For this review, take the finished solid that the model builds, in its own axes (mm). Round coordinates to 2 decimals unless told otherwise and drop trailing zeros. Order: outer loops, then holes, each group sorted by start corner. A loop starts at its lowest first (then second) coordinate and runs counter-clockwise, first axis right, second up. Notation, with made-up numbers: M 3,67 L 57,67 A8 cw 57,77 Z; hole C 16,13 d2. An arc over 180 degrees is marked long. Put each result on its own line as item: value.
from build123d import *

# Parameters (mm, degrees)
SKETCH_8_W           = 73
SKETCH_8_H           = 92
EXTRUDE_5_DEPTH      = 12
SKETCH_9_W           = 71
SKETCH_9_H           = 90
CUT_EXTRUDE_3_DEPTH  = 10
SKETCH_11_W          = 73
SKETCH_11_H          = 6
EXTRUDE_8_DEPTH      = 7
SKETCH_12_W          = 4
SKETCH_12_H          = 19
EXTRUDE_10_DEPTH     = 7
SKETCH_13_W          = 4
SKETCH_13_H          = 21
EXTRUDE_13_DEPTH     = 7
SKETCH_14_W          = 7
SKETCH_14_H          = 12
EXTRUDE_14_DEPTH     = 7
SKETCH_15_W          = 7
SKETCH_15_H          = 58
EXTRUDE_15_DEPTH     = 7
SKETCH_17_W          = 40
SKETCH_17_H          = 6
EXTRUDE_16_DEPTH     = 7
SKETCH_18_W          = 20
SKETCH_18_H          = 5
EXTRUDE_17_DEPTH     = 7
SKETCH_19_W          = 16
SKETCH_19_H          = 4
EXTRUDE_18_DEPTH     = 7
SKETCH_20_W          = 4
SKETCH_20_H          = 7
EXTRUDE_19_DEPTH     = 7
SKETCH_21_W          = 5
SKETCH_21_H          = 31
EXTRUDE_22_DEPTH     = 5
SKETCH_23_W          = 9
SKETCH_23_H          = 12
EXTRUDE_23_DEPTH     = 7
SKETCH_24_W          = 17
SKETCH_24_H          = 10
EXTRUDE_24_DEPTH     = 7
SKETCH_25_W          = 8
SKETCH_25_H          = 4
EXTRUDE_25_DEPTH     = 7
SKETCH_28_W          = 8
SKETCH_28_H          = 31
EXTRUDE_26_DEPTH     = 5
SKETCH_32_W          = 10
SKETCH_32_H          = 1
CUT_EXTRUDE_4_DEPTH  = 5
SKETCH_33_W          = 8
SKETCH_33_H          = 51
EXTRUDE_27_DEPTH     = 5
SKETCH_35_W          = 10
SKETCH_35_H          = 1
EXTRUDE_28_DEPTH     = 10
SKETCH_37_W          = 11
SKETCH_37_H          = 1
CUT_EXTRUDE_7_DEPTH  = 1
SKETCH_39_W          = 11
SKETCH_39_H          = 1
CUT_EXTRUDE_8_DEPTH  = 1
SKETCH_40_W          = 1
SKETCH_40_H          = 1
EXTRUDE_29_DEPTH     = 7
SKETCH_41_R          = 1
CUT_EXTRUDE_9_DEPTH  = 9
EXTRUDE_30_DEPTH     = 4
SKETCH_44_W          = 4
SKETCH_44_H          = 6
SKETCH_44_W_2        = 3
SKETCH_44_H_2        = 5
SKETCH_44_H_3        = 7
SKETCH_44_W_3        = 7
SKETCH_44_H_4        = 7.504780259
EXTRUDE_31_DEPTH     = 7
SKETCH_45_W          = 73
SKETCH_45_H          = 1
CUT_EXTRUDE_10_DEPTH = 100
SKETCH_47_W          = 73
SKETCH_47_H          = 1
CUT_EXTRUDE_11_DEPTH = 100


with BuildPart() as part:
    # 草图8 → 凸台-拉伸5 (new body)
    with BuildSketch(Plane(origin=(0, 0, 0), x_dir=(1, 0, 0), z_dir=(0, 1, 0))):
        with Locations((36.5, 46)):
            Rectangle(SKETCH_8_W, SKETCH_8_H)
    extrude(amount=EXTRUDE_5_DEPTH)

    # 草图9 → 切除-拉伸3 (cut)
    with BuildSketch(Plane(origin=(0, 12, 0), x_dir=(1, 0, 0), z_dir=(0, 1, 0))):
        with Locations((36.5, 46)):
            Rectangle(SKETCH_9_W, SKETCH_9_H)
    extrude(amount=-CUT_EXTRUDE_3_DEPTH, mode=Mode.SUBTRACT)

    # 草图11 → 凸台-拉伸8 (add)
    with BuildSketch(Plane(origin=(0, 0, 0), x_dir=(1, 0, 0), z_dir=(0, 1, 0))):
        with Locations((36.5, 89)):
            Rectangle(SKETCH_11_W, SKETCH_11_H)
    extrude(amount=EXTRUDE_8_DEPTH)

    # 草图12 → 凸台-拉伸10 (add)
    with BuildSketch(Plane(origin=(0, 0, 0), x_dir=(1, 0, 0), z_dir=(0, 1, 0))):
        with Locations((71, 82.5)):
            Rectangle(SKETCH_12_W, SKETCH_12_H)
    extrude(amount=EXTRUDE_10_DEPTH)

    # 草图13 → 凸台-拉伸13 (add)
    with BuildSketch(Plane(origin=(0, 0, 0), x_dir=(1, 0, 0), z_dir=(0, 1, 0))):
        with Locations((2, 81.5)):
            Rectangle(SKETCH_13_W, SKETCH_13_H)
    extrude(amount=EXTRUDE_13_DEPTH)

    # 草图14 → 凸台-拉伸14 (add)
    with BuildSketch(Plane(origin=(0, 0, 0), x_dir=(1, 0, 0), z_dir=(0, 1, 0))):
        with Locations((4.5, 65)):
            Rectangle(SKETCH_14_W, SKETCH_14_H)
    extrude(amount=EXTRUDE_14_DEPTH)

    # 草图15 → 凸台-拉伸15 (add)
    with BuildSketch(Plane(origin=(0, 0, 0), x_dir=(1, 0, 0), z_dir=(0, 1, 0))):
        with Locations((4.5, 30)):
            Rectangle(SKETCH_15_W, SKETCH_15_H)
    extrude(amount=EXTRUDE_15_DEPTH)

    # 草图17 → 凸台-拉伸16 (add)
    with BuildSketch(Plane(origin=(0, 0, 0), x_dir=(1, 0, 0), z_dir=(0, 1, 0))):
        with Locations((21, 27)):
            Rectangle(SKETCH_17_W, SKETCH_17_H)
    extrude(amount=EXTRUDE_16_DEPTH)

    # 草图18 → 凸台-拉伸17 (add)
    with BuildSketch(Plane(origin=(0, 0, 0), x_dir=(1, 0, 0), z_dir=(0, 1, 0))):
        with Locations((11, 47.5)):
            Rectangle(SKETCH_18_W, SKETCH_18_H)
    extrude(amount=EXTRUDE_17_DEPTH)

    # 草图19 → 凸台-拉伸18 (add)
    with BuildSketch(Plane(origin=(0, 0, 0), x_dir=(1, 0, 0), z_dir=(0, 1, 0))):
        with Locations((64, 3)):
            Rectangle(SKETCH_19_W, SKETCH_19_H)
    extrude(amount=EXTRUDE_18_DEPTH)

    # 草图20 → 凸台-拉伸19 (add)
    with BuildSketch(Plane(origin=(0, 0, 0), x_dir=(1, 0, 0), z_dir=(0, 1, 0))):
        with Locations((70, 4.5)):
            Rectangle(SKETCH_20_W, SKETCH_20_H)
    extrude(amount=EXTRUDE_19_DEPTH)

    # 草图21 → 凸台-拉伸22 (add)
    with BuildSketch(Plane(origin=(0, 0, 0), x_dir=(1, 0, 0), z_dir=(0, 1, 0))):
        with Locations((57.5, 28.5)):
            Rectangle(SKETCH_21_W, SKETCH_21_H)
    extrude(amount=EXTRUDE_22_DEPTH)

    # 草图23 → 凸台-拉伸23 (add)
    with BuildSketch(Plane(origin=(0, 0, 0), x_dir=(1, 0, 0), z_dir=(0, 1, 0))):
        with Locations((59.5, 74)):
            Rectangle(SKETCH_23_W, SKETCH_23_H)
    extrude(amount=EXTRUDE_23_DEPTH)

    # 草图24 → 凸台-拉伸24 (add)
    with BuildSketch(Plane(origin=(0, 0, 0), x_dir=(1, 0, 0), z_dir=(0, 1, 0))):
        with Locations((34.5, 73)):
            Rectangle(SKETCH_24_W, SKETCH_24_H)
    extrude(amount=EXTRUDE_24_DEPTH)

    # 草图25 → 凸台-拉伸25 (add)
    with BuildSketch(Plane(origin=(0, 0, 0), x_dir=(1, 0, 0), z_dir=(0, 1, 0))):
        with Locations((17, 73)):
            Rectangle(SKETCH_25_W, SKETCH_25_H)
    extrude(amount=EXTRUDE_25_DEPTH)

    # 草图28 → 凸台-拉伸26 (add)
    with BuildSketch(Plane(origin=(0, 0, 0), x_dir=(1, 0, 0), z_dir=(0, 1, 0))):
        with Locations((37, 28.5)):
            Rectangle(SKETCH_28_W, SKETCH_28_H)
    extrude(amount=EXTRUDE_26_DEPTH)

    # 草图32 → 切除-拉伸4 (cut)
    with BuildSketch(Plane(origin=(0, 12, 0), x_dir=(1, 0, 0), z_dir=(0, 1, 0))):
        with Locations((58, 91.5)):
            Rectangle(SKETCH_32_W, SKETCH_32_H)
    extrude(amount=-CUT_EXTRUDE_4_DEPTH, mode=Mode.SUBTRACT)

    # 草图33 → 凸台-拉伸27 (add)
    with BuildSketch(Plane(origin=(0, 0, 0), x_dir=(1, 0, 0), z_dir=(0, 1, 0))):
        with Locations((17, 38.5)):
            Rectangle(SKETCH_33_W, SKETCH_33_H)
    extrude(amount=EXTRUDE_27_DEPTH)

    # 草图35 → 凸台-拉伸28 (add)
    with BuildSketch(Plane(origin=(0, 12, 0), x_dir=(1, 0, 0), z_dir=(0, 1, 0))):
        with Locations((58, 91.5)):
            Rectangle(SKETCH_35_W, SKETCH_35_H)
    extrude(amount=-EXTRUDE_28_DEPTH)

    # 草图37 → 切除-拉伸7 (cut)
    with BuildSketch(Plane(origin=(0, 12, 0), x_dir=(1, 0, 0), z_dir=(0, 1, 0))):
        with Locations((58.5, 91.5)):
            Rectangle(SKETCH_37_W, SKETCH_37_H)
    extrude(amount=-CUT_EXTRUDE_7_DEPTH, mode=Mode.SUBTRACT)

    # 草图39 → 切除-拉伸8 (cut)
    with BuildSketch(Plane(origin=(0, 8, 0), x_dir=(1, 0, 0), z_dir=(0, 1, 0))):
        with Locations((58.5, 91.5)):
            Rectangle(SKETCH_39_W, SKETCH_39_H)
    extrude(amount=CUT_EXTRUDE_8_DEPTH, mode=Mode.SUBTRACT)

    # 草图40 → 凸台-拉伸29 (add)
    with BuildSketch(Plane(origin=(0, 0, 0), x_dir=(1, 0, 0), z_dir=(0, 1, 0))):
        with Locations((4.5, 85.5)):
            Rectangle(SKETCH_40_W, SKETCH_40_H)
    extrude(amount=EXTRUDE_29_DEPTH)

    # 草图41 → 切除-拉伸9 (cut)
    with BuildSketch(Plane(origin=(0, 12, 0), x_dir=(1, 0, 0), z_dir=(0, 1, 0))):
        with Locations((4, 5)):
            Circle(SKETCH_41_R)
        with Locations((70, 6)):
            Circle(SKETCH_41_R)
        with Locations((70, 87)):
            Circle(SKETCH_41_R)
        with Locations((4, 87)):
            Circle(SKETCH_41_R)
    extrude(amount=-CUT_EXTRUDE_9_DEPTH, mode=Mode.SUBTRACT)

    # 草图42 → 凸台-拉伸30 (add)
    with BuildSketch(Plane(origin=(0, 12, 0), x_dir=(1, 0, 0), z_dir=(0, 1, 0))):
        Polygon((53, 92), (53, 91), (1, 91), (1, 1), (72, 1), (72, 91), (64, 91), (64, 92), (73, 92), (73, 0), (0, 0), (0, 92), align=None)
    extrude(amount=EXTRUDE_30_DEPTH)

    # 草图44 → 凸台-拉伸31 (add)
    with BuildSketch(Plane(origin=(0, 0, 0), x_dir=(1, 0, 0), z_dir=(0, 1, 0))):
        with Locations((3, 88)):
            Rectangle(SKETCH_44_W, SKETCH_44_H)
        with Locations((70.5, 88.5)):
            Rectangle(SKETCH_44_W_2, SKETCH_44_H_2)
        with Locations((70, 4.5)):
            Rectangle(SKETCH_44_W, SKETCH_44_H_3)
        with Locations((4.5, 4.75239013)):
            Rectangle(SKETCH_44_W_3, SKETCH_44_H_4)
    extrude(amount=EXTRUDE_31_DEPTH)

    # 草图45 → 切除-拉伸10 (cut)
    with BuildSketch(Plane.XY):
        with Locations((36.5, 0.5)):
            Rectangle(SKETCH_45_W, SKETCH_45_H)
    extrude(amount=-CUT_EXTRUDE_10_DEPTH, mode=Mode.SUBTRACT)

    # 草图47 → 切除-拉伸11 (cut)
    with BuildSketch(Plane.XY):
        with Locations((36.5, 15.5)):
            Rectangle(SKETCH_47_W, SKETCH_47_H)
    extrude(amount=-CUT_EXTRUDE_11_DEPTH, mode=Mode.SUBTRACT)


solid = part.part
(1) Add section A-A on y = 3.5. State how many separate pieces and enclosed holes the cut face has, then the cut area to 3 significant figures.
A:
separate pieces: 5
enclosed holes: 2
area: 2,580 mm2
(2) To check wall thickness, follow L1, parallel to Z at x = 36.5, y = 2.5; L2, parallel to X at y = 4.25, z = -14; L3, parallel to X at y = 13, z = -46. State the ranges of each line that lie inside material, in increasing order.
A:
L1: z = -92 to -86, -78 to -68, -44 to -13, -1 to 0
L2: x = 0 to 8, 13 to 21, 33 to 41, 55 to 60, 72 to 73
L3: x = 0 to 1, 72 to 73
(3) Add section D-D on x = 12. Give the boundary of the cut face in (y, z), then the cut area to 3 significant figures.
A:
outline: M 1,-92 L 15,-92 L 15,-91 L 7,-91 L 7,-86 L 2,-86 L 2,-50 L 7,-50 L 7,-45 L 2,-45 L 2,-30 L 7,-30 L 7,-24 L 2,-24 L 2,-1 L 15,-1 L 15,0 L 1,0 Z
area: 198 mm2
(4) Add section C-C on z = -19. Give the boundary of the cut face in (x, y), then the cut area to 3 significant figures.
A:
outline: M 0,1 L 73,1 L 73,15 L 72,15 L 72,2 L 60,2 L 60,5 L 55,5 L 55,2 L 41,2 L 41,5 L 33,5 L 33,2 L 21,2 L 21,5 L 13,5 L 13,2 L 8,2 L 8,7 L 1,7 L 1,15 L 0,15 Z
area: 197 mm2
(5) Add section B-B on x = 48. Give the boundary of the cut face in (y, z), then the cut area to 3 significant figures.
A:
outline: M 1,-92 L 15,-92 L 15,-91 L 7,-91 L 7,-86 L 2,-86 L 2,-1 L 15,-1 L 15,0 L 1,0 Z
area: 143 mm2
(6) Insertion check: pin 1 Ø1 at (x, z) = (41, -81) entering from +Y; pin 2 Ø12 at (x, z) = (34, -11.5) entering from +Y; pin 3 Ø2 at (x, z) = (68, -5) entering from +Y. Each pin has a flat end and moves straight along its axis. Give the tip position at first contact, or say it passes through.
A:
pin 1: stops at y = 2
pin 2: stops at y = 5
pin 3: stops at y = 7
